Design review of the part shown in the three views and the two pictorial views. Dimensions are in mm from the part's minimum x, y and z. A direction names the side the tool comes from. Round coordinates to 2 decimals unless told otherwise and drop trailing zeros. Write each loop counter-clockwise with the first axis right and the second up, starting at its lowest first coordinate (ties: lowest second). Pieces come first, ordered by that corner, then holes. Notation, with made-up numbers: (23, -21.75) - (50, -21.75) arc R31 ccw to (50, 5.25) - close; hole circle Ø10 at (80.25, 76). An arc over 180 degrees is marked (long way). One line per item, written item: value. Start each with the question number.
Q1. For probe 1 along X at (y, z) = (21.75, 152.4); probe 2 along X at (y, z) = (23.75, 61); probe 3 along Z at (x, y) = (340, 23.75), list the stretches that pass through material, from the lowest coordinate up.
Q2. Add section A-A on y = 20. Give the number of separate pieces and of enclosed holes in the cut face, and give its area (3 significant figures).
Q3. Mouldability with a two-part tool opening along X and no side actions: class the marked faces 3 and 4 as +X half, -X half, draft (parallel to the pull), parting line (faces both ways), or undercut.
Q4. Clearance check with a flat-ended pin moving along its axis: pin 1 Ø3 at (x, z) = (171, 164.5) entering from +Y. State where the tip first meets the part, or that it passes through.
Q5. Tool access review of the marked faces 1 and 2: name each direction out of +Z, -Z, +X, -X, +Y, -Y from which nothing blocks a thin tool from reaching the whole face with its end or side.
Q6. Add section D-D on x = 73. Write out the cut boundary in (y, z).
Q7. Add section C-C on z = 50.8. Write out the cut boundary in (x, y).
Q8. Add section B-B on x = 355.6. Write out the cut boundary in (y, z).
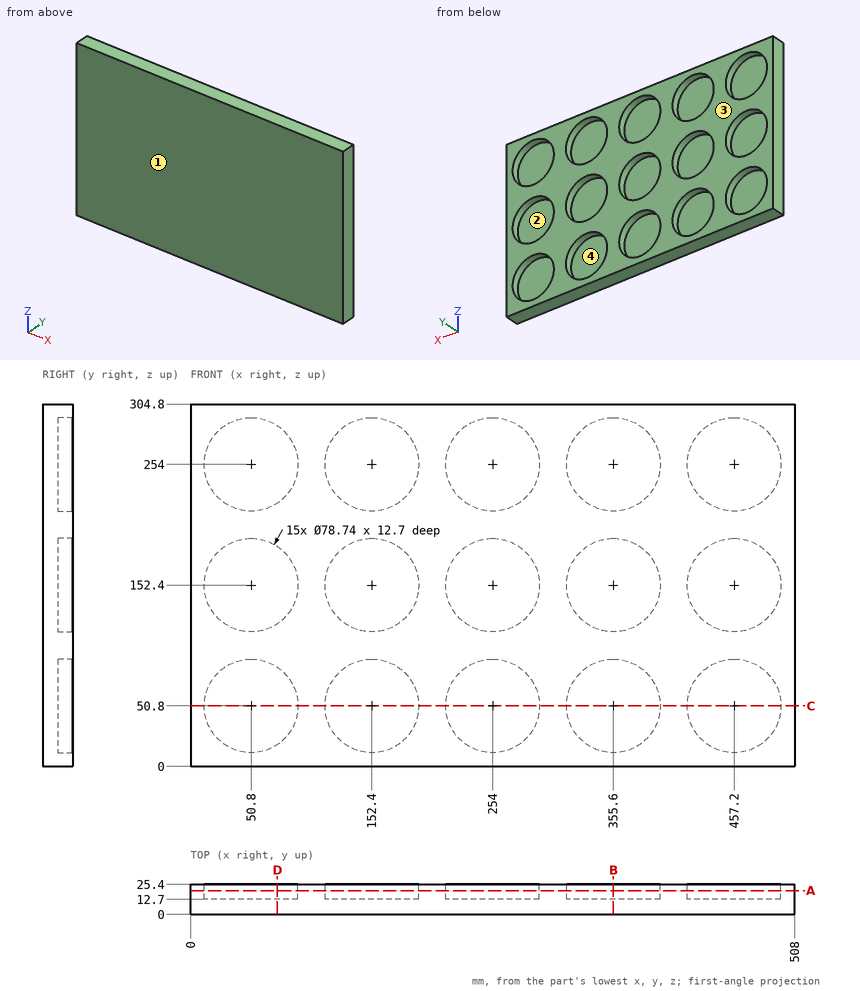
Result set:
1. probe 1: x = 0 to 11.43, 90.17 to 113.03, 191.77 to 214.63, 293.37 to 316.23, 394.97 to 417.83, 496.57 to 508
1. probe 2: x = 0 to 12.77, 88.83 to 114.37, 190.43 to 215.97, 292.03 to 317.57, 393.63 to 419.17, 495.23 to 508
1. probe 3: z = 0 to 14.65, 86.95 to 116.25, 188.55 to 217.85, 290.15 to 304.8
2. separate pieces: 1
2. enclosed holes: 15
2. area: 81,800 mm^2
3. face 3: draft
3. face 4: undercut
4. pin 1: stops at y = 12.7
5. face 1: +Z, -Z, +X, -X, -Y
5. face 2: +Y
6. outline: (0, 0) - (25.4, 0) - (25.4, 18.29) - (12.7, 18.29) - (12.7, 83.31) - (25.4, 83.31) - (25.4, 119.89) - (12.7, 119.89) - (12.7, 184.91) - (25.4, 184.91) - (25.4, 221.49) - (12.7, 221.49) - (12.7, 286.51) - (25.4, 286.51) - (25.4, 304.8) - (0, 304.8) - close
7. outline: (0, 0) - (508, 0) - (508, 25.4) - (496.57, 25.4) - (496.57, 12.7) - (417.83, 12.7) - (417.83, 25.4) - (394.97, 25.4) - (394.97, 12.7) - (316.23, 12.7) - (316.23, 25.4) - (293.37, 25.4) - (293.37, 12.7) - (214.63, 12.7) - (214.63, 25.4) - (191.77, 25.4) - (191.77, 12.7) - (113.03, 12.7) - (113.03, 25.4) - (90.17, 25.4) - (90.17, 12.7) - (11.43, 12.7) - (11.43, 25.4) - (0, 25.4) - close
8. outline: (0, 0) - (25.4, 0) - (25.4, 11.43) - (12.7, 11.43) - (12.7, 90.17) - (25.4, 90.17) - (25.4, 113.03) - (12.7, 113.03) - (12.7, 191.77) - (25.4, 191.77) - (25.4, 214.63) - (12.7, 214.63) - (12.7, 293.37) - (25.4, 293.37) - (25.4, 304.8) - (0, 304.8) - close
